from build123d import *

# Parameters (mm, degrees)
SKETCH1_W           = 29
SKETCH1_H           = 29
BOSS_EXTRUDE1_DEPTH = 30
SKETCH2_R           = 1
CUT_EXTRUDE1_DEPTH  = 2.5
SKETCH3_R           = 1.5
CUT_EXTRUDE2_DEPTH  = 2.8
SKETCH4_R           = 1.5
CUT_EXTRUDE3_DEPTH  = 2.5
SKETCH5_R           = 1
CUT_EXTRUDE4_DEPTH  = 2
SKETCH6_R           = 13.85
BOSS_EXTRUDE2_DEPTH = 12.6
SKETCH7_R           = 16.7
BOSS_EXTRUDE3_DEPTH = 43
FILLET1_R           = 0.3
SKETCH8_R           = 13.25
CUT_EXTRUDE5_DEPTH  = 11.5


with BuildPart() as part:
    # Sketch1 → Boss-Extrude1 (new body)
    with BuildSketch(Plane.XY):
        with Locations((14.5, 14.5)):
            Rectangle(SKETCH1_W, SKETCH1_H)
    extrude(amount=BOSS_EXTRUDE1_DEPTH)

    # Sketch2 → Cut-Extrude1 (cut)
    with BuildSketch(Plane(origin=(0, 29, 0), x_dir=(1, 0, 0), z_dir=(0, 1, 0))):
        with Locations(Location((8.5, -28, 0), (0, 0, 270))):
            Circle(SKETCH2_R)
        with Locations(Location((20.5, -28, 0), (0, 0, 90))):
            Circle(SKETCH2_R)
    extrude(amount=-CUT_EXTRUDE1_DEPTH, mode=Mode.SUBTRACT)

    # Sketch3 → Cut-Extrude2 (cut)
    with BuildSketch(Plane.XZ):
        with Locations(Location((24.5, 27, 0), (0, 0, 270))):
            Circle(SKETCH3_R)
        with Locations(Location((4.5, 27, 0), (0, 0, 90))):
            Circle(SKETCH3_R)
    extrude(amount=-CUT_EXTRUDE2_DEPTH, mode=Mode.SUBTRACT)

    # Sketch4 → Cut-Extrude3 (cut)
    with BuildSketch(Plane.XZ):
        with Locations(Location((14.5, 3.3, 0), (0, 0, 270))):
            Circle(SKETCH4_R)
    extrude(amount=-CUT_EXTRUDE3_DEPTH, mode=Mode.SUBTRACT)

    # Sketch5 → Cut-Extrude4 (cut)
    with BuildSketch(Plane.XZ):
        with Locations(Location((20.5, 25.3, 0), (0, 0, 270))):
            Circle(SKETCH5_R)
        with Locations(Location((20.5, 3.3, 0), (0, 0, 270))):
            Circle(SKETCH5_R)
        with Locations(Location((8.5, 3.3, 0), (0, 0, 90))):
            Circle(SKETCH5_R)
        with Locations(Location((8.5, 25.3, 0), (0, 0, 90))):
            Circle(SKETCH5_R)
    extrude(amount=-CUT_EXTRUDE4_DEPTH, mode=Mode.SUBTRACT)

    # Sketch6 → Boss-Extrude2 (add)
    with BuildSketch(Plane.XY.offset(30)):
        with Locations((14.5, 14.5)):
            Circle(SKETCH6_R)
    extrude(amount=BOSS_EXTRUDE2_DEPTH)

    # Sketch7 → Boss-Extrude3 (add)
    with BuildSketch(Plane.XY.offset(42.6)):
        with Locations((14.5, 14.5)):
            Circle(SKETCH7_R)
    extrude(amount=BOSS_EXTRUDE3_DEPTH)

    # Fillet1
    fillet1_edges = [part.edges().sort_by_distance(p)[0] for p in [
        (29, 14.5, 30),
        (14.5, 29, 30),
        (0, 14.5, 30),
        (14.5, 29, 0),
        (0.65, 14.5, 30),
        (29, 14.5, 0),
        (14.5, 0, 0),
        (0, 14.5, 0),
        (14.5, 0, 30),
        (0, 29, 15),
        (29, 29, 15),
        (29, 0, 15),
        (0, 0, 15),
    ]]
    fillet(fillet1_edges, radius=FILLET1_R)

    # Sketch8 → Cut-Extrude5 (cut)
    with BuildSketch(Plane.XY.offset(85.6)):
        with Locations((14.5, 14.5)):
            Circle(SKETCH8_R)
    extrude(amount=-CUT_EXTRUDE5_DEPTH, mode=Mode.SUBTRACT)


solid = part.part
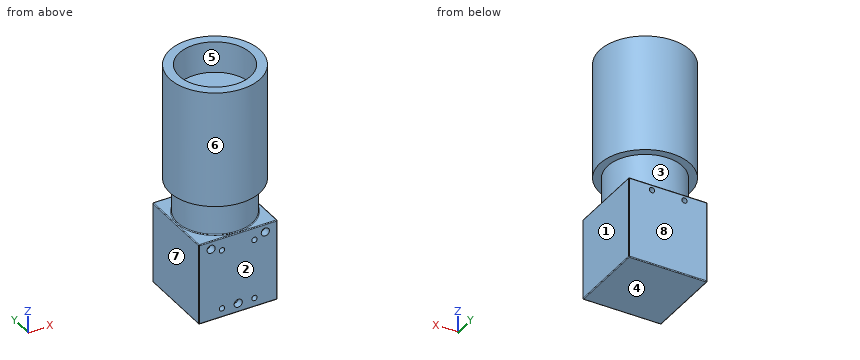
Work out the finished part from the listing and answer in its coordinate system (mm). Face numbers are marked on the shaded views. A direction names the side the tool comes from. Give positions to 0.01 mm unless a question says otherwise; leave off trailing zeros. Order: outer loops, then holes, each group sorted by start corner. A loop starts at its lowest first (then second) coordinate and runs counter-clockwise, first axis right, second up. Notation, with made-up numbers: (64.5, 49) -> (72.5, 49) arc R30 cw to (72.5, 88) -> close; hole circle Ø9 at (25.5, 1.25). An arc over 180 degrees is marked (long way). One line per item, written item: value.
Item 1: Flat-ended cylindrical pins translate along their axes: P1, Ø10, axis at y = 4.5, z = 33, coming from the -X side; P2, Ø0.9, axis at x = 15, z = 3, coming from the -Y side; P3, Ø8, axis at y = 4.5, z = 75, coming from the +X side; P4, Ø8, axis at x = 6.5, y = 20, coming from the +Z side. Find the tip coordinate at first contact, or state that the pin passes through.
Answer sheet:
P1: x = 0
P2: y = 2.5
P3: x = 30.08
P4: z = 85.6
Item 2: Straight lines are drawn through the part: probe 1 along X at (y, z) = (1.25, 3.3); probe 2 along X at (y, z) = (0.4, 25.3); probe 3 along Z at (x, y) = (8.5, 0.6). For each, find the intervals that lie inside material, in ascending order.
Answer sheet:
probe 1: 0 to 7.5, 9.5 to 13, 16 to 19.5, 21.5 to 29
probe 2: 0 to 7.5, 9.5 to 19.5, 21.5 to 29
probe 3: 0 to 2.3, 4.3 to 24.3, 26.3 to 30, 42.6 to 85.6
Item 3: Find section D-D, the plane z = 52. Give the vertices of the cut face in (x, y), plus the area to 3 significant figures.
Answer sheet:
outline: circle Ø33.4 at (14.5, 14.5)
area: 876 mm²
Item 4: Find section B-B, the plane x = 14.5. Give the vertices of the cut face in (y, z).
Answer sheet:
outline: (-2.2, 42.6) -> (0.65, 42.6) -> (0.65, 30.3) arc R0.3 cw to (0.35, 30) -> (0.3, 30) arc R0.3 ccw to (0, 29.7) -> (0, 4.8) -> (2.5, 4.8) -> (2.5, 1.8) -> (0, 1.8) -> (0, 0.3) arc R0.3 ccw to (0.3, 0) -> (28.7, 0) arc R0.3 ccw to (29, 0.3) -> (29, 29.7) arc R0.3 ccw to (28.7, 30) -> (28.65, 30) arc R0.3 cw to (28.35, 30.3) -> (28.35, 42.6) -> (31.2, 42.6) -> (31.2, 85.6) -> (27.75, 85.6) -> (27.75, 74.1) -> (1.25, 74.1) -> (1.25, 85.6) -> (-2.2, 85.6) -> close
Item 5: A tool of negligible diameter and unlimited length cuts with its end or side. For the marked faces 1, 2, 3 and 4, from which of +Z, -Z, +X, -X, +Y, -Y can it reach the whole face along a straight path? Write none if from no direction.
Answer sheet:
face 1: -Z, +X, +Y, -Y
face 2: -Z, +X, -X, -Y
face 3: none
face 4: -Z, +X, -X, +Y, -Y
Item 6: Find section C-C, the plane z = 41.5. Give the vertices of the cut face in (x, y).
Answer sheet:
outline: circle Ø27.7 at (14.5, 14.5)
Item 7: Find section A-A, the plane z = 9. Give the vertices of the cut face in (x, y), plus the area to 3 significant figures.
Answer sheet:
outline: (0, 0.3) arc R0.3 ccw to (0.3, 0) -> (28.7, 0) arc R0.3 ccw to (29, 0.3) -> (29, 28.7) arc R0.3 ccw to (28.7, 29) -> (0.3, 29) arc R0.3 ccw to (0, 28.7) -> close
area: 841 mm²
Item 8: Determine the mould class of the marked faces 5, 6, 7 and 8 for opening direction Y: released by +Y, released by -Y, zero draft, split by the parting line, or undercut.
Answer sheet:
face 5: undercut
face 6: split by the parting line
face 7: zero draft
face 8: released by +Y
